```python
from build123d import *

# Parameters (mm, degrees)
SKETCH1_W            = 40
SKETCH1_H            = 70
SKETCH1_R            = 7.5
BOSS_EXTRUDE1_DEPTH  = 6.35
M5_CLEARANCE_HOLE1_D = 5.5
CHAMFER1_SIZE        = 10


with BuildPart() as part:
    # Sketch1 → Boss-Extrude1 (new body)
    with BuildSketch(Plane.XY):
        Rectangle(SKETCH1_W, SKETCH1_H)
        with Locations((0, 20)):
            Circle(SKETCH1_R, mode=Mode.SUBTRACT)
    extrude(amount=BOSS_EXTRUDE1_DEPTH)

    # M5 Clearance Hole1 (through all)
    with Locations(Plane.XY.offset(6.35)):
        with Locations((0, -10), (0, -25)):
            Hole(M5_CLEARANCE_HOLE1_D / 2)

    # Chamfer1
    chamfer1_edges = [part.edges().sort_by_distance(p)[0] for p in [
        (-20, 35, 3.175),
        (20, 35, 3.175),
        (20, -35, 3.175),
        (-20, -35, 3.175),
    ]]
    chamfer(chamfer1_edges, length=CHAMFER1_SIZE)


solid = part.part
```
Could you check a few things on this model? Use its own coordinates, in mm. Coordinates: 2 decimals unless noted, no trailing zeros. Loops run counter-clockwise (first coordinate to the right, second up) from the corner with the lowest first, then second, coordinate; pieces in that order, holes last.
1) Please list where these lines run through material, in increasing order: line 1 along Y through (x, z) = (0, 3); line 2 along X through (y, z) = (-7.5, 2); line 3 along X through (y, z) = (-11, 4).
Reported:
line 1: y = -35 to -27.75, -22.25 to -12.75, -7.25 to 12.5, 27.5 to 35
line 2: x = -20 to -1.15, 1.15 to 20
line 3: x = -20 to -2.56, 2.56 to 20
2) Imagine slicing it at A-A (y = -10). List the corners of the cut face in (x, z) for me.
Reported:
outline: (-20, 0) - (-2.75, 0) - (-2.75, 6.35) - (-20, 6.35) - close; (2.75, 0) - (20, 0) - (20, 6.35) - (2.75, 6.35) - close
3) Thinking about a two-plate mould opening in X: for faces 1 (the face through (0.358, -22.273, 3.131)), 2 (the face through (2.027, -8.141, 3.131)), 3 (the face through (0, 0, 0)), 4 (the face through (20, 0, 3)), which applies, released by +X, released by -X, zero draft, split by the parting line, or undercut?
Reported:
face 1: undercut
face 2: undercut
face 3: zero draft
face 4: released by +X
4) Imagine slicing it at B-B (z = 4.5). List the corners of the cut face in (x, y) for me.
Reported:
outline: (-20, -25) - (-10, -35) - (10, -35) - (20, -25) - (20, 25) - (10, 35) - (-10, 35) - (-20, 25) - close; hole circle Ø15 at (0, 20); hole circle Ø5.5 at (0, -25); hole circle Ø5.5 at (0, -10)
5) Will these pins go through, and if not, where does the flat tip stop? pin 1 Ø1 at (x, y) = (-12.5, -13) entering from -Z; pin 2 Ø3.5 at (x, y) = (0, -10) entering from -Z; pin 3 Ø1 at (x, z) = (-12.5, 4) entering from -Y.
Reported:
pin 1: stops at z = 0
pin 2: passes through
pin 3: stops at y = -33
6) Imagine slicing it at D-D (x = -11.5). List the corners of the cut face in (y, z) for me, and give its area (3 significant figures).
Reported:
outline: (-33.5, 0) - (33.5, 0) - (33.5, 6.35) - (-33.5, 6.35) - close
area: 425 mm2
7) Imagine slicing it at C-C (x = 3.5). List the corners of the cut face in (y, z) for me, and give its area (3 significant figures).
Reported:
outline: (-35, 0) - (13.37, 0) - (13.37, 6.35) - (-35, 6.35) - close; (26.63, 0) - (35, 0) - (35, 6.35) - (26.63, 6.35) - close
area: 360 mm2
